Geometry: final body of the model. Coordinates: model frame, mm. Give positions to 0.01 mm unless a question says otherwise; leave off trailing zeros. Loops run counter-clockwise (first coordinate to the right, second up) from the corner with the lowest first, then second, coordinate; pieces in that order, holes last. Notation, with made-up numbers: (30.25, 57.25) - (80.25, 57.25) arc R26 ccw to (80.25, 71.25) - close; hole circle Ø2 at (45, 11.25). An arc over 180 degrees is marked (long way). Use one line per item in the form item = value.
```python
from build123d import *

# Parameters (mm, degrees)
F0_R     = 34.5
F1_DEPTH = 2
F0_R_2   = 36
F2_DEPTH = 9
F4_R     = 2


# Not quite as in the source:
# - a fillet or chamfer that OpenCascade refuses, or shapes differently, is made with other operations: its cross-section is extruded or revolved along the edge and cut away or added


with BuildPart() as f1:
    # F0 (on Top) → F1 (new body)
    with BuildSketch(Plane.XY):
        Circle(F0_R)
    extrude(amount=F1_DEPTH)

    # F0 (on Top) → F2 (join)
    with BuildSketch(Plane.XY):
        Circle(F0_R_2)
        Circle(F0_R, mode=Mode.SUBTRACT)
    extrude(amount=F2_DEPTH)

    # F3: fillet of radius 2 on 2 edges, made by hand

    # F3_s1 → F3_t2 (revolve)
    with BuildSketch(Plane.XZ):
        with BuildLine():
            ThreePointArc((34.5, 4), (33.9142135624, 2.5857864376), (32.5, 2))
            Line((32.5, 2), (34.5, 2))
            Line((34.5, 2), (34.5, 4))
        make_face()
    revolve(axis=Axis((0, 0, 2), (0, 0, 1)))

    # F3_s3 → F3_t4 (revolve, cut)
    with BuildSketch(Plane.XZ):
        with BuildLine():
            ThreePointArc((36, 9), (34.9188611699, 8.2882531983), (34.5, 7.0635083269))
            Line((34.5, 7.0635083269), (34.5, 9))
            Line((34.5, 9), (36, 9))
        make_face()
    revolve(axis=Axis((0, 0, 9), (0, 0, 1)), mode=Mode.SUBTRACT)

    # F4
    f4_edges = [f1.edges().sort_by_distance(p)[0] for p in [
        (-36, 0, 0),
    ]]
    fillet(f4_edges, radius=F4_R)


solid = f1.part
```
(1) Pull-direction query (Y, two-part tool) for faces 1 (the face through (0, 0, 2)), 2 (the face through (-4.686, 35.694, 5.451)), 3 (the face through (0, 0, 0)); classes: released by +Y, released by -Y, zero draft, split by the parting line, or undercut.
Solution:
face_1 = undercut
face_2 = split by the parting line
face_3 = zero draft
(2) Material intervals for L1, parallel to Y at x = 0, z = 5.1; L2, parallel to X at y = -1, z = 6.5; L3, parallel to Z at x = -15, y = 19, sorted ascending. Write a range as from..to.
Solution:
L1 = -36..-34.5, 34.5..36
L2 = -35.99..-34.49, 34.49..35.99
L3 = 0..2
(3) Pin query (flat end, axial travel): P1, Ø1, axis at y = -6.5, z = 3.5, coming from the +X side; P2, Ø3, axis at y = -14, z = 6.5, coming from the +X side; P3, Ø1, axis at x = 26, z = 3.5, coming from the -Y side. Return the tip coordinate at first contact, or that it passes through.
Solution:
P1 = 35.5
P2 = 33.76
P3 = -25.41
(4) Cut plane D-D (z = 1). Return the cut outline in (x, y), plus the area to 3 significant figures.
Solution:
outline = circle Ø71.46 at (0, 0)
area = 4,010 mm2
(5) Cut plane B-B (z = 6). Return the cut outline in (x, y), plus the area to 3 significant figures.
Solution:
outline = circle Ø72 at (0, 0); hole circle Ø69 at (0, 0)
area = 332 mm2
(6) Cut plane A-A (y = 0). Return the cut outline in (x, z).
Solution:
outline = (-36, 2) arc R2 ccw to (-34, 0) - (34, 0) arc R2 ccw to (36, 2) - (36, 9) arc R2 ccw to (34.5, 7.06) - (34.5, 4) arc R2 cw to (32.5, 2) - (-32.5, 2) arc R2 cw to (-34.5, 4) - (-34.5, 7.06) arc R2 ccw to (-36, 9) - close
